```python
from build123d import *

# Parameters (mm, degrees)
F0_R      = 22
F0_R_2    = 17
F1_DEPTH  = 6
F0_R_3    = 8
F2_DEPTH  = 40
F6_DEPTH  = 80
F7_R      = 6
F8_DEPTH  = 20
F9_W      = 25
F9_H      = 6
F10_DEPTH = 100
F12_DEPTH = 6
F14_DEPTH = 6


with BuildPart() as f1:
    # F0 (on Top) → F1 (new body)
    with BuildSketch(Plane.XY):
        Circle(F0_R)
        Circle(F0_R_2, mode=Mode.SUBTRACT)
    extrude(amount=F1_DEPTH)

    # F0 (on Top) → F2 (join)
    with BuildSketch(Plane.XY):
        Circle(F0_R_2)
        Circle(F0_R_3, mode=Mode.SUBTRACT)
    extrude(amount=F2_DEPTH)


with BuildPart() as f3_1:
    # F3: instance of F1
    add(f1.part.mirror(Plane.XY.offset(40)))


with BuildPart() as f1_1:
    add(f1.part)

    # F5: union F3_1
    add(f3_1.part)

    # F4 (on Top) → F6 (join, through all)
    with BuildSketch(Plane.XY):
        Polygon((-16.7332005307, 3), (-21.7944947177, 3), (-99.7944947177, 3), (-99.7944947177, -3), (-21.7944947177, -3), (-16.7332005307, -3), align=None)
    extrude(amount=F6_DEPTH)

    # F7 (on face) → F8 (join)
    with BuildSketch(Plane(origin=(-99.7944947177, 0, 0), x_dir=(0, -1, 0), z_dir=(-1, 0, 0))):
        with BuildLine():
            Line((38, 80), (3, 80))
            Line((3, 80), (3, 44))
            Line((3, 44), (28, 44))
            Line((28, 44), (28, 38))
            Line((28, 38), (3, 38))
            Line((3, 38), (3, 0))
            Line((3, 0), (-3, 0))
            Line((-3, 0), (-3, 38))
            Line((-3, 38), (-28, 38))
            Line((-28, 38), (-28, 44))
            Line((-28, 44), (-3, 44))
            Line((-3, 44), (-3, 80))
            Line((-3, 80), (-38, 80))
            Line((-38, 80), (-38, 44))
            Line((-38, 44), (-16, -20))
            ThreePointArc((-16, -20), (0, -36), (16, -20))
            Line((16, -20), (38, 44))
            Line((38, 44), (38, 80))
        make_face()
        with Locations((0, -20)):
            Circle(F7_R, mode=Mode.SUBTRACT)
        with Locations((-22, 62)):
            Circle(F7_R, mode=Mode.SUBTRACT)
        with Locations((22, 62)):
            Circle(F7_R, mode=Mode.SUBTRACT)
    extrude(amount=-F8_DEPTH)

    # F9 (on face) → F10 (join)
    with BuildSketch(Plane(origin=(-99.7944947177, 0, 0), x_dir=(0, -1, 0), z_dir=(-1, 0, 0))):
        with Locations((-15.5, 41)):
            Rectangle(F9_W, F9_H)
        with Locations((15.5, 41)):
            Rectangle(F9_W, F9_H)
    extrude(amount=-F10_DEPTH)

    # F11 (on face) → F12 (cut, through all)
    with BuildSketch(Plane.XY.offset(44)):
        Polygon((0.2055052823, -16.9987578246), (-79.7944947177, -28), (0.2055052823, -28), align=None)
    extrude(amount=-F12_DEPTH, mode=Mode.SUBTRACT)

    # F13 (on face) → F14 (cut, through all)
    with BuildSketch(Plane.XY.offset(44)):
        Polygon((0.2055052823, 28), (-79.7944947177, 28), (0.2055052823, 16.9987578246), align=None)
    extrude(amount=-F14_DEPTH, mode=Mode.SUBTRACT)


solid = f1_1.part
```
Geometry: final body of the model. Coordinates: model frame, mm. A direction names the side the tool comes from. Round coordinates to 2 decimals unless told otherwise and drop trailing zeros. Loops run counter-clockwise (first coordinate to the right, second up) from the corner with the lowest first, then second, coordinate; pieces in that order, holes last.
Item 1: Contact query for flat-ended pins moving along their axis: P1, Ø12, axis at x = -61.5, z = 26.5, coming from the +Y side; P2, Ø5, axis at x = -56.5, z = 21.5, coming from the -Y side; P3, Ø7.5, axis at x = -53, y = -21, coming from the -Z side; P4, Ø9.5, axis at y = 0, z = -20, coming from the +X side. Output: stop coordinate, or through.
Checked values:
P1: stops at y = 3
P2: stops at y = -3
P3: stops at z = 38
P4: passes through
Item 2: Reachability of faces 1 (the flat face through (-79.794, 9, 36)), 2 (the flat face through (-4, -3, 41)), 3 (the cylindrical face through (-89.93, 26.42, 66.06)) from +Z, -Z, +X, -X, +Y, -Y: full face, straight path, thin tool, end or side. Return the list, or none.
Checked values:
face 1: none
face 2: +Z, -Z
face 3: -X
Item 3: Line query: L1, parallel to Z at x = -10, y = 14.5; L2, parallel to Y at x = 0, z = 49; L3, parallel to Z at x = -93, y = 0. Output: solid intervals per line, ascending.
Checked values:
L1: z = 0 to 6, 38 to 44, 74 to 80
L2: y = -17 to -8, 8 to 17
L3: z = -36 to -26, -14 to 80
Item 4: Section B-B, the plane x = -89.5. Output: boundary loops of the cut face in (y, z), plus the area to 3 significant figures.
Checked values:
outline: (-38, 44) - (-16, -20) arc R16 ccw to (16, -20) - (38, 44) - (38, 80) - (-38, 80) - close; hole circle Ø12 at (-22, 62); hole circle Ø12 at (0, -20); hole circle Ø12 at (22, 62)
area: 6,250 mm2
Item 5: Mould query, pull axis X, two halves, no side actions, for faces 4 (the flat face through (-49, 13, 38)), 5 (the flat face through (-49, -3, 62)), 6 (the flat face through (-7, 5, 0)), 7 (the flat face through (-99.794, 1, 36)). Classes: released by +X, released by -X, zero draft, split by the parting line, or undercut.
Checked values:
face 4: undercut
face 5: undercut
face 6: zero draft
face 7: released by -X
Item 6: Section A-A, the plane z = 62. Output: boundary loops of the cut face in (x, y), plus the area to 3 significant figures.
Checked values:
outline: (-99.79, -38) - (-79.79, -38) - (-79.79, -28) - (-99.79, -28) - close; (-99.79, -16) - (-79.79, -16) - (-79.79, -3) - (-16.73, -3) arc R17 ccw (long way) to (-16.73, 3) - (-79.79, 3) - (-79.79, 16) - (-99.79, 16) - close; (-99.79, 28) - (-79.79, 28) - (-79.79, 38) - (-99.79, 38) - close; hole circle Ø16 at (0, 0)
area: 2,120 mm2
Item 7: Section C-C, the plane y = 18.5. Output: boundary loops of the cut face in (x, z), plus the area to 3 significant figures.
Checked values:
outline: (-99.79, -12.73) - (-79.79, -12.73) - (-79.79, 38) - (-10.71, 38) - (-10.71, 44) - (-79.79, 44) - (-79.79, 57.13) - (-99.79, 57.13) - close; (-99.79, 66.87) - (-79.79, 66.87) - (-79.79, 80) - (-99.79, 80) - close; (-11.91, 0) - (11.91, 0) - (11.91, 6) - (-11.91, 6) - close; (-11.91, 74) - (11.91, 74) - (11.91, 80) - (-11.91, 80) - close
area: 2,360 mm2
Item 8: Section D-D, the plane x = 2. Output: boundary loops of the cut face in (y, z).
Checked values:
outline: (-21.91, 0) - (-7.75, 0) - (-7.75, 80) - (-21.91, 80) - (-21.91, 74) - (-16.88, 74) - (-16.88, 6) - (-21.91, 6) - close; (7.75, 0) - (21.91, 0) - (21.91, 6) - (16.88, 6) - (16.88, 74) - (21.91, 74) - (21.91, 80) - (7.75, 80) - close
